Design review of the part built by this model. Coordinates are the model's own, in mm. A direction names the side the tool comes from. Coordinates: 2 decimals unless noted, no trailing zeros. One line per question, with ' | ' between items.
from build123d import *

# Parameters (mm, degrees)
BOSS_EXTRUDE1_DEPTH = 250


with BuildPart() as part:
    # Sketch1 → Boss-Extrude1 (new body)
    with BuildSketch(Plane(origin=(0, 0, -150), x_dir=(-1, 0, 0), z_dir=(0, 0, -1))):
        with BuildLine():
            Line((-14.999999999, 12.999999999), (-14.999999999, 10.499999999))
            Line((-14.999999999, 10.499999999), (-14.499999999, 9.999999999))
            Line((-14.499999999, 9.999999999), (-14.999999999, 9.5))
            Line((-14.999999999, 9.5), (-14.999999999, 4.5))
            Line((-14.999999999, 4.5), (-14.5, 4.5))
            Line((-14.5, 4.5), (-14.5, 4))
            Line((-14.5, 4), (-12.200000005, 4))
            Line((-12.200000005, 4), (-12.200000005, 7.999999995))
            ThreePointArc((-12.200000005, 7.999999995), (-11.582683434, 8.923879532), (-10.492893215, 8.70710678))
            Line((-10.492893215, 8.70710678), (-6, 4.214213564))
            Line((-6, 4.214213564), (-6, 0.312520903))
            Line((-6, 0.312520903), (-5.7, 0))
            Line((-5.7, 0), (-6, -0.312520901))
            Line((-6, -0.312520901), (-6, -4.214213564))
            Line((-6, -4.214213564), (-10.492893215, -8.70710678))
            ThreePointArc((-10.492893215, -8.70710678), (-11.582683434, -8.923879532), (-12.200000005, -7.999999995))
            Line((-12.200000005, -7.999999995), (-12.200000005, -4))
            Line((-12.200000005, -4), (-14.5, -4))
            Line((-14.5, -4), (-14.5, -4.5))
            Line((-14.5, -4.5), (-14.999999999, -4.5))
            Line((-14.999999999, -4.5), (-14.999999999, -9.500000003))
            Line((-14.999999999, -9.500000003), (-14.499999999, -10.000000002))
            Line((-14.499999999, -10.000000002), (-14.999999999, -10.500000001))
            Line((-14.999999999, -10.500000001), (-14.999999999, -13))
            ThreePointArc((-14.999999999, -13), (-14.414213561, -14.414213562), (-12.999999999, -15))
            Line((-12.999999999, -15), (-10.5, -15))
            Line((-10.5, -15), (-10.000000001, -14.500000001))
            Line((-10.000000001, -14.500000001), (-9.500000001, -15))
            Line((-9.500000001, -15), (-4.5, -15))
            Line((-4.5, -15), (-4.5, -14.5))
            Line((-4.5, -14.5), (-4, -14.5))
            Line((-4, -14.5), (-4, -12.200000005))
            Line((-4, -12.200000005), (-7.999999995, -12.200000005))
            ThreePointArc((-7.999999995, -12.200000005), (-8.923879532, -11.582683434), (-8.70710678, -10.492893215))
            Line((-8.70710678, -10.492893215), (-4.214213564, -6))
            Line((-4.214213564, -6), (-0.312520903, -6))
            Line((-0.312520903, -6), (0, -5.7))
            Line((0, -5.7), (0.312520901, -6))
            Line((0.312520901, -6), (4.214213564, -6))
            Line((4.214213564, -6), (8.70710678, -10.492893215))
            ThreePointArc((8.70710678, -10.492893215), (8.923879532, -11.582683434), (7.999999995, -12.200000005))
            Line((7.999999995, -12.200000005), (4, -12.200000005))
            Line((4, -12.200000005), (4, -14.5))
            Line((4, -14.5), (4.5, -14.5))
            Line((4.5, -14.5), (4.5, -15))
            Line((4.5, -15), (9.500000001, -15))
            Line((9.500000001, -15), (9.989897949, -14.5))
            Line((9.989897949, -14.5), (10.489897949, -15))
            Line((10.489897949, -15), (13, -15))
            ThreePointArc((13, -15), (14.414213562, -14.414213562), (15, -13))
            Line((15, -13), (15, -10.5))
            Line((15, -10.5), (14.500000001, -10.000000001))
            Line((14.500000001, -10.000000001), (15, -9.500000001))
            Line((15, -9.500000001), (15, -4.5))
            Line((15, -4.5), (14.5, -4.5))
            Line((14.5, -4.5), (14.5, -4))
            Line((14.5, -4), (12.200000005, -4))
            Line((12.200000005, -4), (12.200000005, -7.999999995))
            ThreePointArc((12.200000005, -7.999999995), (11.582683434, -8.923879532), (10.492893215, -8.70710678))
            Line((10.492893215, -8.70710678), (6, -4.214213564))
            Line((6, -4.214213564), (6, -0.312520903))
            Line((6, -0.312520903), (5.7, 0))
            Line((5.7, 0), (6, 0.312520901))
            Line((6, 0.312520901), (6, 4.214213564))
            Line((6, 4.214213564), (10.492893215, 8.707106779))
            ThreePointArc((10.492893215, 8.707106779), (11.582683434, 8.923879532), (12.200000005, 7.999999994))
            Line((12.200000005, 7.999999994), (12.200000005, 4))
            Line((12.200000005, 4), (14.5, 4))
            Line((14.5, 4), (14.5, 4.5))
            Line((14.5, 4.5), (15, 4.5))
            Line((15, 4.5), (15, 9.500000001))
            Line((15, 9.500000001), (14.500000001, 10.000000001))
            Line((14.500000001, 10.000000001), (15, 10.5))
            Line((15, 10.5), (15, 12.999999999))
            ThreePointArc((15, 12.999999999), (14.414213562, 14.414213561), (13, 14.999999999))
            Line((13, 14.999999999), (10.500000001, 14.999999999))
            Line((10.500000001, 14.999999999), (10.000000002, 14.499999999))
            Line((10.000000002, 14.499999999), (9.500000003, 14.999999999))
            Line((9.500000003, 14.999999999), (4.5, 14.999999999))
            Line((4.5, 14.999999999), (4.5, 14.5))
            Line((4.5, 14.5), (4, 14.5))
            Line((4, 14.5), (4, 12.200000005))
            Line((4, 12.200000005), (7.999999995, 12.200000005))
            ThreePointArc((7.999999995, 12.200000005), (8.923879532, 11.582683434), (8.70710678, 10.492893215))
            Line((8.70710678, 10.492893215), (4.214213564, 6))
            Line((4.214213564, 6), (0.312520903, 6))
            Line((0.312520903, 6), (0, 5.7))
            Line((0, 5.7), (-0.312520901, 6))
            Line((-0.312520901, 6), (-4.214213564, 6))
            Line((-4.214213564, 6), (-8.707106779, 10.492893215))
            ThreePointArc((-8.707106779, 10.492893215), (-8.923879532, 11.582683434), (-7.999999994, 12.200000005))
            Line((-7.999999994, 12.200000005), (-4, 12.200000005))
            Line((-4, 12.200000005), (-4, 14.5))
            Line((-4, 14.5), (-4.5, 14.5))
            Line((-4.5, 14.5), (-4.5, 14.999999999))
            Line((-4.5, 14.999999999), (-9.5, 14.999999999))
            Line((-9.5, 14.999999999), (-9.999999999, 14.499999999))
            Line((-9.999999999, 14.499999999), (-10.499999999, 14.999999999))
            Line((-10.499999999, 14.999999999), (-12.999999999, 14.999999999))
            ThreePointArc((-12.999999999, 14.999999999), (-14.414213561, 14.414213561), (-14.999999999, 12.999999999))
        make_face()
        with BuildLine():
            Line((4.808326112, 3.676955262), (2.902349714, 1.770978864))
            ThreePointArc((2.902349714, 1.770978864), (3.4, 0), (2.902349714, -1.770978864))
            Line((2.902349714, -1.770978864), (4.808326112, -3.676955262))
            Line((4.808326112, -3.676955262), (3.676955262, -4.808326112))
            Line((3.676955262, -4.808326112), (1.770978864, -2.902349714))
            ThreePointArc((1.770978864, -2.902349714), (0, -3.4), (-1.770978864, -2.902349714))
            Line((-1.770978864, -2.902349714), (-3.676955262, -4.808326112))
            Line((-3.676955262, -4.808326112), (-4.808326112, -3.676955262))
            Line((-4.808326112, -3.676955262), (-2.902349714, -1.770978864))
            ThreePointArc((-2.902349714, -1.770978864), (-3.4, 0), (-2.902349714, 1.770978864))
            Line((-2.902349714, 1.770978864), (-4.808326112, 3.676955262))
            Line((-4.808326112, 3.676955262), (-3.676955262, 4.808326112))
            Line((-3.676955262, 4.808326112), (-1.770978864, 2.902349714))
            ThreePointArc((-1.770978864, 2.902349714), (0, 3.4), (1.770978864, 2.902349714))
            Line((1.770978864, 2.902349714), (3.676955262, 4.808326112))
            Line((3.676955262, 4.808326112), (4.808326112, 3.676955262))
        make_face(mode=Mode.SUBTRACT)
    extrude(amount=-BOSS_EXTRUDE1_DEPTH)


solid = part.part
Q1. For pin 1 (1.2 mm diameter, centred on x = 3, z = -37.5, fed in from +Y); pin 2 (1.5 mm diameter, centred on x = 1, y = 1, fed in from -Z); pin 3 (1.8 mm diameter, centred on x = 13.5, z = -26, fed in from -Y); pin 4 (0.6 mm diameter, centred on x = 4, z = -84, fed in from +Y), all flat-tipped, find the tip position at first contact; note any pin that passes through.
Returned:
pin 1: stops at y = 6 | pin 2: passes through | pin 3: stops at y = -15 | pin 4: stops at y = 14.5
Q2. Tool access review of faces 1 (the flat face through (-8.215, 6.429, -26.75)), 2 (the flat face through (15, -7, -27)): name each direction out of +Z, -Z, +X, -X, +Y, -Y from which nothing blocks a thin tool from reaching the whole face with its end or side.
Returned:
face 1: +Z, -Z | face 2: +Z, -Z, +X, +Y, -Y
Q3. Draft analysis for pull direction Y (two halves, no side actions). For faces 3 (the flat face through (-7, -15, -27)), 4 (the flat face through (6, -2, -27)), 5 (the flat face through (-15, 7, -27)), state which applies: +Y half, -Y half, draft (parallel to the pull), parting line (faces both ways), or undercut.
Returned:
face 3: -Y half | face 4: undercut | face 5: draft
Q4. To check wall thickness, follow line 1 along Y through (x, z) = (-1.75, 88.5); line 2 along X through (y, z) = (-3.5, -20.5); line 3 along X through (y, z) = (7.25, -61). State the ranges of each line that lie inside material, in increasing order.
Returned:
line 1: y = -6 to -2.92, 2.92 to 6 | line 2: x = -6 to -4.63, -2.37 to 2.37, 4.63 to 6 | line 3: x = -15 to -12.2, -9.04 to -5.46, 5.46 to 9.04, 12.2 to 15
